Source: CAD feature listing. Evaluate the final solid. Frame: model axes, mm. A direction names the side the tool comes from. Give positions to 0.01 mm unless a question says otherwise; leave off trailing zeros. Order: outer loops, then holes, each group sorted by start corner. A loop starts at its lowest first (then second) coordinate and runs counter-clockwise, first axis right, second up.
Autodesk Inventor part; units mm, degrees
ref_plane "YZ Plane" through (0, 0, 0) normal (1, 0, 0) x (0, 1, 0)
ref_plane "XZ Plane" through (0, 0, 0) normal (0, 1, 0) x (-1, 0, 0)
ref_plane "XY Plane" through (0, 0, 0) normal (0, 0, 1) x (1, 0, 0)
sketch "Sketch1" plane through (0, 0, 0) normal (0, 1, 0) x (-1, 0, 0)
  circle A0 centre (0, 0) radius 2.6
  line L0 (0, 0) -> (2.6, 0) construction
  circle A1 centre (20, 0) radius 2.6
  circle A2 centre (22, -31) radius 2.6
  line L1 (22, -31) -> (24.6, -31) construction
  line L2 (22, -31) -> (22, -33.6) construction
  circle A3 centre (40, -31) radius 2.6
  circle A4 centre (22, -77) radius 2.6
  circle A5 centre (40, -77) radius 2.6
  circle A6 centre (20, -108) radius 2.6
  circle A7 centre (0, -108) radius 2.6
  circle A8 centre (20, 0) radius 8.95 construction
  circle A9 centre (0, 0) radius 8.95 construction
  circle A10 centre (20, -108) radius 8.95 construction
  circle A11 centre (0, -108) radius 8.95 construction
  circle A12 centre (40, -31) radius 5.775 construction
  circle A13 centre (40, -77) radius 5.775 construction
  line L3 (27.9103, 4.1868) -> (45.1042, -28.2985)
  line L4 (45.1042, -79.7015) -> (27.9103, -112.1868)
  line L5 (-8.95, 0) -> (-8.95, -108)
  line L6 (20, 8.95) -> (0, 8.95)
  line L7 (20, -116.95) -> (0, -116.95)
  line L8 (45.775, -31) -> (45.775, -77)
  arc A14 (45.1042, -79.7015) -> (45.775, -77) centre (40, -77) ccw
  arc A15 (45.775, -31) -> (45.1042, -28.2985) centre (40, -31) ccw
  arc A16 (27.9103, 4.1868) -> (20, 8.95) centre (20, 0) ccw
  arc A17 (0, 8.95) -> (-8.95, 0) centre (0, 0) ccw
  arc A18 (-8.95, -108) -> (0, -116.95) centre (0, -108) ccw
  arc A19 (20, -116.95) -> (27.9103, -112.1868) centre (20, -108) ccw
  point P0 (42.6, -31)
  point P1 (40, -33.6)
  point P2 (24.6, -77)
  point P3 (22, -79.6)
  point P4 (42.6, -77)
  point P5 (40, -79.6)
  dimension "d0" = 5.2
  dimension "d1" = 20
  dimension "d2" = 31
  dimension "d3" = 22
  dimension "d6" = 18
  dimension "d9" = 46
  dimension "d12" = 31
  dimension "d13" = 6.35
  dimension "d14" = 3.175
extrude "Extrusion1" add sketch "Sketch1" along normal blind 4.7625
sketch "Sketch2" plane through (0, 4.7625, 0) normal (0, 1, 0) x (1, 0, 0)
  arc A0 (0, -8.95) -> (8.95, 0) centre (0, 0) ccw
  line L0 (8.95, 0) -> (8.95, 108)
  arc A1 (8.95, 108) -> (0, 116.95) centre (0, 108) ccw
  line L1 (0, 116.95) -> (-20, 116.95)
  arc A2 (-20, 116.95) -> (-27.9103, 112.1868) centre (-20, 108) ccw
  line L2 (-27.9103, 112.1868) -> (-45.1042, 79.7015)
  arc A3 (-45.1042, 79.7015) -> (-45.775, 77) centre (-40, 77) ccw
  line L3 (-45.775, 77) -> (-45.775, 31)
  arc A4 (-45.775, 31) -> (-45.1042, 28.2985) centre (-40, 31) ccw
  line L4 (-45.1042, 28.2985) -> (-27.9103, -4.1868)
  arc A5 (-27.9103, -4.1868) -> (-20, -8.95) centre (-20, 0) ccw
  line L5 (-20, -8.95) -> (0, -8.95)
  circle A6 centre (-20, 0) radius 2.6
  circle A7 centre (-22, 31) radius 2.6
  circle A8 centre (-40, 31) radius 2.6
  circle A9 centre (-22, 77) radius 2.6
  circle A10 centre (-40, 77) radius 2.6
  circle A11 centre (-20, 108) radius 2.6
  circle A12 centre (0, 108) radius 2.6
  circle A13 centre (0, 0) radius 2.6
  circle A14 centre (-40, 54) radius 9
  point P0 (-45.775, 60.9029)
  point P1 (-45.775, 47.0971)
  dimension "d17" = 18
  dimension "d18" = 46
  dimension "d19" = 23
extrude "Extrusion2" cut sketch "Sketch2" against normal through all contours L3 A14 picked at (-38.3999, 55.6279)
fillet "Fillet1" radius 6.35 2 edges at (-45.775, 2.3813, -47.0971) (-45.775, 2.3813, -60.9029)
sketch "Sketch3" plane through (0, 4.7625, 0) normal (0, 1, 0) x (1, 0, 0)
  line L0 (-45.1042, 28.2985) -> (-27.9103, -4.1868)
  line L1 (-35.9749, 11.05) -> (-30, 11.05)
  line L2 (-30, 11.05) -> (-30, -0.2387)
  line L3 (-20, -8.95) -> (0, -8.95)
  line L4 (-27.9103, 112.1868) -> (-45.1042, 79.7015)
  line L5 (-35.9749, 96.95) -> (-30, 96.95)
  line L6 (-30, 96.95) -> (-30, 108.2387)
  circle A0 centre (-20, 0) radius 2.6
  point P0 (0, 0)
  dimension "d23" = 20
  dimension "d24" = 10
extrude "Extrusion3" cut sketch "Sketch3" against normal through all contours L1 L2 L0 | L6 L5 L4
fillet "Fillet2" radius 1.5875 6 edges at (-30, 2.3813, -11.05) (-30, 2.3813, 0.2387) (-35.9749, 2.3813, -11.05) (-35.9749, 2.3813, -96.95) (-30, 2.3813, -96.95) (-30, 2.3813, -108.2387)
equation "\"d12\" = d2"
equation "\"d19\" = 0.5 * d18"
properties part number "CNC-001-StructureGusset2" material "Steel AISI 1008 91 HR"
1) Section query B-B on y = 3.2. State how many separate pieces and enclosed holes the cut face has, and give its area (3 significant figures).
Checks:
separate pieces: 1
enclosed holes: 8
area: 5,580 mm2
2) First-contact query: pin 1 Ø1 at (x, y) = (-33.5, 2.5) entering from -Z; pin 2 Ø1.7 at (x, y) = (-33.5, 2) entering from +Z. Flat tips, straight axial feed; report the tip coordinate or a pass-through.
Checks:
pin 1: stops at z = -96.95
pin 2: stops at z = -11.05
3) Section query A-A on x = -41.5. Output: boundary loops of the cut face in (y, z).
Checks:
outline: (0, -86.51) - (4.76, -86.51) - (4.76, -79.12) - (0, -79.12) - close; (0, -74.88) - (4.76, -74.88) - (4.76, -63.34) - (0, -63.34) - close; (0, -44.66) - (4.76, -44.66) - (4.76, -33.12) - (0, -33.12) - close; (0, -28.88) - (4.76, -28.88) - (4.76, -21.49) - (0, -21.49) - close
4) Ray query, L1, parallel to Z at x = 0, y = 1.1; L2, parallel to Z at x = -20, y = 2.95; L3, parallel to Z at x = -22, y = 3.05. Return the intervals inside material, ascending.
Checks:
L1: z = -116.95 to -110.6, -105.4 to -2.6, 2.6 to 8.95
L2: z = -116.95 to -110.6, -105.4 to -78.66, -75.34 to -32.66, -29.34 to -2.6, 2.6 to 8.95
L3: z = -116.72 to -109.66, -106.34 to -79.6, -74.4 to -33.6, -28.4 to -1.66, 1.66 to 8.72
5) Section query D-D on z = -84.5. Output: boundary loops of the cut face in (x, y).
Checks:
outline: (-42.56, 0) - (8.95, 0) - (8.95, 4.76) - (-42.56, 4.76) - close
6) Section query C-C on z = -54. Output: boundary loops of the cut face in (x, y).
Checks:
outline: (-31, 0) - (8.95, 0) - (8.95, 4.76) - (-31, 4.76) - close
7) Reachability of faces 1 (the face through (8.95, 2, -53)), 2 (the face through (-30, 2, -5)) from +Z, -Z, +X, -X, +Y, -Y: full face, straight path, thin tool, end or side. Return the list, or none.
Checks:
face 1: +Z, -Z, +X, +Y, -Y
face 2: +Z, -X, +Y, -Y
8) Pull-direction query (Z, two-part tool) for faces 3 (the face through (-10, 2, 8.95)), 4 (the face through (-45.775, 2, -35)), 5 (the face through (-44.045, 2.348, -43.017)); classes: +Z half, -Z half, draft (parallel to the pull), parting line (faces both ways), or undercut.
Checks:
face 3: +Z half
face 4: draft
face 5: undercut
